Geometry check sheet. Reference: drawing and pictorial views, mm from the part's lowest x, y, z. A direction names the side the tool comes from. Round coordinates to 2 decimals unless told otherwise and drop trailing zeros. Order: outer loops, then holes, each group sorted by start corner. A loop starts at its lowest first (then second) coordinate and runs counter-clockwise, first axis right, second up. Notation, with made-up numbers: (18, -10) -> (43, -10) arc R19 cw to (43, 12) -> close; hole circle Ø8 at (48.5, 31). An arc over 180 degrees is marked (long way). Return JSON: item names as keys, results as strings. Group by question number.
1) Scan lines: L1, parallel to Y at x = 20, z = 2; L2, parallel to Y at x = 20, z = 6; L3, parallel to Z at x = 36, y = 10.5. Record each from-to range of solid material in increasing order.
2) Section check D-D on y = 4. Enter the section's corners in (x, z).
3) Depth check by flat-ended pin: pin 1 (6 mm diameter, centred on x = 20, z = 5, fed in from -Y); pin 2 (10 mm diameter, centred on x = 20, y = 20, fed in from -Z) (3 decimals); pin 3 (5 mm diameter, centred on y = 29, z = 5.5, fed in from -X); pin 4 (1 mm diameter, centred on x = 16, z = 5, fed in from -Y). Enter the tip coordinate at first touch or a pass-through.
4) Tool access check on the marked faces 1 and 2. Record the directions out of +Z, -Z, +X, -X, +Y, -Y that give a thin tool (end or side, any length) a straight path to the whole face; none if there is none.
5) Section check C-C on z = 2.5. Enter the section's corners in (x, y), plus the area to 3 significant figures.
6) Section check A-A on y = 20. Enter the section's corners in (x, z).
7) Draft check along Y on the marked faces 3, 4 and 5. Enter one of: pulls with the +Y half, pulls with the -Y half, needs draft (parallel to the pull), parting line crosses it, or undercut.
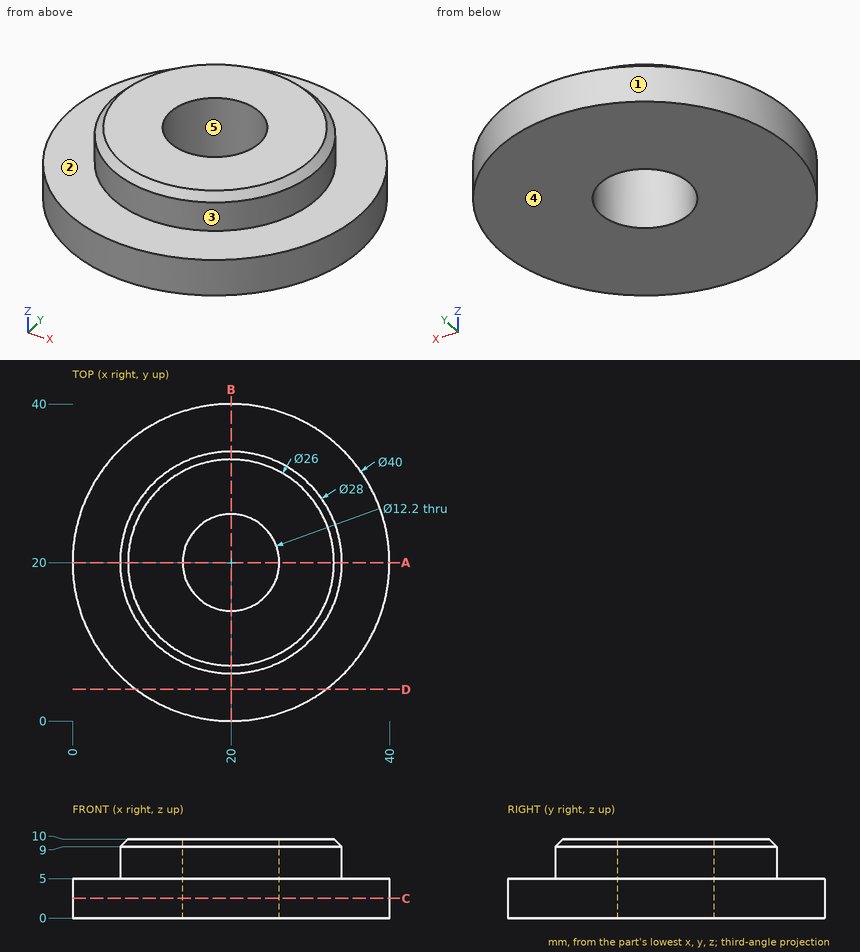
Check result:
{
 "1": {"L1": "0 to 13.9, 26.1 to 40", "L2": "6 to 13.9, 26.1 to 34", "L3": "0 to 5"},
 "2": {"outline": "(8, 0) -> (32, 0) -> (32, 5) -> (8, 5) -> close"},
 "3": {"pin 1": "y = 0", "pin 2": "through", "pin 3": "x = 1.1", "pin 4": "y = 0.31"},
 "4": {"face 1": "+Z, -Z", "face 2": "+Z"},
 "5": {"outline": "circle Ø40 at (20, 20); hole circle Ø12.2 at (20, 20)", "area": "1,140 mm^2"},
 "6": {"outline": "(0, 0) -> (13.9, 0) -> (13.9, 10) -> (7, 10) -> (6, 9) -> (6, 5) -> (0, 5) -> close; (26.1, 0) -> (40, 0) -> (40, 5) -> (34, 5) -> (34, 9) -> (33, 10) -> (26.1, 10) -> close"},
 "7": {"face 3": "parting line crosses it", "face 4": "needs draft", "face 5": "undercut"}
}
